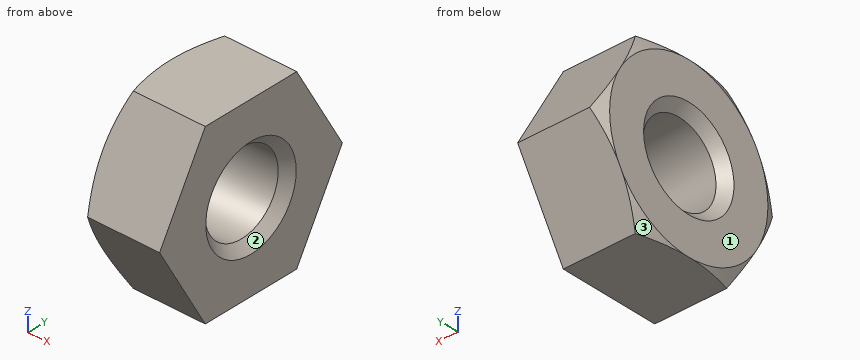
Autodesk Inventor part; units mm, degrees
ref_plane "cp_XY" through (1.6, 0, 0) normal (1, 0, 0) x (0, 0, -1)
ref_plane "cp_YZ" through (1.6, 0, 0) normal (0, 0, -1) x (0, 1, 0)
ref_plane "cp_ZX" through (1.6, 0, 0) normal (0, 1, 0) x (1, 0, 0)
sketch "Sketch_1" plane through (0, 0, 0) normal (0, 0, 1) x (1, 0, 0)
  line L0 (1.6, 0) -> (-1.6, 0)
  line L1 (-1.6, 0) -> (-1.6, 3.5)
  line L2 (-1.6, 3.5) -> (-1.2825, 4.05)
  line L3 (-1.2825, 4.05) -> (1.6, 4.05)
  line L4 (1.6, 4.05) -> (1.6, 0)
  line L5 (1.6, 0) -> (-1.6, 0)
revolve "Revolution1" add sketch "Sketch_1" angle 360 about axis through (1.6, 0, 0) along (1, 0, 0)
sketch "Sketch_2" plane through (0, 0, 0) normal (0, 0, 1) x (1, 0, 0)
  line L0 (1.6, 0) -> (-1.6, 0)
  line L1 (-1.6, 0) -> (-1.6, 2)
  line L2 (-1.6, 2) -> (-1.221, 1.621)
  line L3 (-1.221, 1.621) -> (1.221, 1.621)
  line L4 (1.221, 1.621) -> (1.6, 2)
  line L5 (1.6, 2) -> (1.6, 0)
  line L6 (1.6, 0) -> (-1.6, 0)
revolve "Revolution2" cut sketch "Sketch_2" angle 360 about axis through (1.6, 0, 0) along (1, 0, 0)
thread "Thread1"
sketch "Sketch_3" plane through (0, 0, 0) normal (1, 0, 0) x (0, 1, 0)
  line L0 (-7, 7) -> (-7, -7)
  line L1 (-7, -7) -> (7, -7)
  line L2 (7, -7) -> (7, 7)
  line L3 (7, 7) -> (-7, 7)
  line L4 (-2.0207, 3.5) -> (-4.0415, 0)
  line L5 (-4.0415, 0) -> (-2.0207, -3.5)
  line L6 (-2.0207, -3.5) -> (2.0207, -3.5)
  line L7 (2.0207, -3.5) -> (4.0415, 0)
  line L8 (4.0415, 0) -> (2.0207, 3.5)
  line L9 (2.0207, 3.5) -> (-2.0207, 3.5)
extrude "Extrusion1" cut sketch "Sketch_3" along normal mid plane 3.2
ref_plane "cp_XY" through (1.6, 0, 0) normal (1, 0, 0) x (0, 0, -1)
ref_plane "cp_YZ" through (1.6, 0, 0) normal (0, 0, -1) x (0, 1, 0)
ref_plane "cp_ZX" through (1.6, 0, 0) normal (0, 1, 0) x (1, 0, 0)
ref_plane "nut_to_screw_XY" through (0, 0, 0) normal (1, 0, 0) x (0, 0, -1)
ref_plane "nut_to_screw_YZ" through (0, 0, 0) normal (0, 0, -1) x (0, 1, 0)
ref_plane "nut_to_screw_ZX" through (0, 0, 0) normal (0, 1, 0) x (1, 0, 0)
properties part number "LBNR4" material "鋼、炭素鋼"
For this review, take the finished solid that the model builds, in its own axes (mm). Face numbers are marked on the shaded views. Coordinates: 2 decimals unless noted, no trailing zeros. Write each loop counter-clockwise with the first axis right and the second up, starting at its lowest first coordinate (ties: lowest second). Pieces come first, ordered by that corner, then holes. Notation, with made-up numbers: (71, -29.75) - (92, -29.75) arc R19 cw to (92, -18.75) - close; hole circle Ø5 at (71.25, -1). An arc over 180 degrees is marked (long way). Put each result on its own line as item: value.
1. Add section B-B, the plane x = -0.8. Give the boundary of the cut face in (y, z).
Values found:
outline: (-4.04, 0) - (-2.02, -3.5) - (2.02, -3.5) - (4.04, 0) - (2.02, 3.5) - (-2.02, 3.5) - close; hole circle Ø3.24 at (0, 0)
2. Mouldability with a two-part tool opening along Z and no side actions: class the marked faces 1, 2 and 3 as released by +Z, released by -Z, zero draft, split by the parting line, or undercut.
Values found:
face 1: zero draft
face 2: undercut
face 3: released by -Z
3. Wall thickness on probe 1 along Z at (x, y) = (0.35, 0); probe 2 along Z at (x, y) = (-1.4, -0.5); probe 3 along Y at (x, z) = (0.25, 0.25): over which ranges is each line inside the solid? List them lowest first.
Values found:
probe 1: -3.5 to -1.62, 1.62 to 3.5
probe 2: -3.5 to -1.73, 1.73 to 3.5
probe 3: -3.9 to -1.6, 1.6 to 3.9
4. Add section A-A, the plane x = 1.45. Give the boundary of the cut face in (y, z).
Values found:
outline: (-4.04, 0) - (-2.02, -3.5) - (2.02, -3.5) - (4.04, 0) - (2.02, 3.5) - (-2.02, 3.5) - close; hole circle Ø3.7 at (0, 0)
